Autodesk Inventor part; units mm, degrees
ref_plane "YZ Plane" through (0, 0, 0) normal (1, 0, 0) x (0, 1, 0)
ref_plane "XZ Plane" through (0, 0, 0) normal (0, 1, 0) x (-1, 0, 0)
ref_plane "XY Plane" through (0, 0, 0) normal (0, 0, 1) x (1, 0, 0)
sketch "Sketch1" plane through (0, 0, 0) normal (0, 0, 1) x (1, 0, 0)
  circle A0 centre (0, 0) radius 12.35
  circle A1 centre (7.4246, 7.4246) radius 12.2
  line L0 (-13.413, -13.413) -> (25.4094, 25.4094) construction
  line L1 (-10.6165, 0) -> (15.2552, 0) construction
  line L2 (7.4246, 7.4246) -> (15.8638, 6.41) construction
  line L3 (16.6649, 18.5138) -> (22.6753, 24.5242) construction
  circle A2 centre (15.8638, 6.41) radius 1.5
  line L4 (7.4246, 7.4246) -> (-1.0146, 8.4392) construction
  circle A3 centre (-1.0146, 8.4392) radius 1.5
  line L5 (0, 0) -> (-1.0146, 8.4392) construction
  line L6 (0, 0) -> (1.0146, -8.4392) construction
  circle A4 centre (1.0146, -8.4392) radius 1.5
  circle A5 centre (-9.8288, -9.8288) radius 12.2
  line L7 (-5.2409, -11.1828) -> (0, 0)
  point P0 (11.6813, -4.0087)
  point P1 (-0.7603, -1.6223)
  dimension "d0" = 24.7
  dimension "d1" = 24.4
  dimension "d2" = 0
  dimension "d3" = 45
  dimension "d4" = 0
  dimension "d5" = 10.5
  dimension "d20" = 8.5
  dimension "d21" = 3
  dimension "d22" = 3
  dimension "d23" = 3
  dimension "d24" = 24.4
  dimension "d25" = 24.4
  dimension "d26" = 4.5
extrude "Extrusion1" add sketch "Sketch1" along normal blind 3 contours A0 A5 A4 L7 A1 | A0 L7 A5 A4
sketch "Sketch3" plane through (0, 0, 3) normal (0, 0, 1) x (1, 0, 0)
  circle A0 centre (0, 0) radius 12.35
  circle A1 centre (7.4246, 7.4246) radius 12.2
  line L0 (-13.413, -13.413) -> (25.4094, 25.4094) construction
  line L1 (-10.6165, 0) -> (15.2552, 0) construction
  line L2 (7.4246, 7.4246) -> (15.8638, 6.41) construction
  line L3 (16.6649, 18.5138) -> (22.6753, 24.5242) construction
  circle A2 centre (15.8638, 6.41) radius 1.5
  line L4 (7.4246, 7.4246) -> (-1.0146, 8.4392) construction
  circle A3 centre (-1.0146, 8.4392) radius 1.5
  line L5 (0, 0) -> (-1.0146, 8.4392) construction
  line L6 (0, 0) -> (1.0146, -8.4392) construction
  circle A4 centre (1.0146, -8.4392) radius 1.5
  circle A5 centre (-9.8288, -9.8288) radius 12.2
  line L7 (-5.2409, -11.1828) -> (0, 0)
  point P0 (11.6813, -4.0087)
  point P1 (-0.7603, -1.6223)
  point P2 (-0.7743, -1.6522)
  point P3 (2.1356, -7.4425)
  point P4 (2.3507, -9.1211)
  point P5 (2.146, -12.1621)
  dimension "d32" = 24.7
  dimension "d33" = 24.4
  dimension "d34" = 0
  dimension "d35" = 45
  dimension "d36" = 0
  dimension "d37" = 10.5
  dimension "d38" = 8.5
  dimension "d39" = 3
  dimension "d40" = 3
  dimension "d41" = 3
  dimension "d42" = 24.4
  dimension "d43" = 24.4
  dimension "d44" = 4.5
extrude "Extrusion3" add sketch "Sketch3" along normal blind 15.5 contours A0 A5 A4 L7 A1 | A4 A5 picked at (2.3363, -8.2121)
sketch "Sketch4" plane through (0, 0, 3) normal (0, 0, 1) x (1, 0, 0)
  line L0 (-2.1493, -8.7099) -> (-0.8017, -5.8346)
  line L1 (-0.8017, -5.8346) -> (2.3621, -5.5639)
  line L2 (2.3621, -5.5639) -> (4.1785, -8.1686)
  line L3 (4.1785, -8.1686) -> (2.8309, -11.0439)
  line L4 (2.8309, -11.0439) -> (-0.3329, -11.3146)
  line L5 (-0.3329, -11.3146) -> (-2.1493, -8.7099)
  point P0 (0, 0)
  point P1 (1.0146, -8.4392)
  dimension "d49" = 5.5
extrude "Extrusion4" cut sketch "Sketch4" along normal blind 2 and the other way blind 1
sketch "Sketch5" plane through (0, 0, 18.5) normal (0, 0, 1) x (1, 0, 0)
  circle A0 centre (0, 0) radius 12.35
  circle A1 centre (7.4246, 7.4246) radius 12.2
  line L0 (-13.413, -13.413) -> (25.4094, 25.4094) construction
  line L1 (-10.6165, 0) -> (15.2552, 0) construction
  line L2 (7.4246, 7.4246) -> (15.8638, 6.41) construction
  line L3 (16.6649, 18.5138) -> (22.6753, 24.5242) construction
  circle A2 centre (15.8638, 6.41) radius 1.5
  line L4 (7.4246, 7.4246) -> (-1.0146, 8.4392) construction
  circle A3 centre (-1.0146, 8.4392) radius 1.5
  line L5 (0, 0) -> (-1.0146, 8.4392) construction
  line L6 (0, 0) -> (1.0146, -8.4392) construction
  circle A4 centre (1.0146, -8.4392) radius 1.5
  circle A5 centre (-9.8288, -9.8288) radius 12.2
  line L7 (-5.2409, -11.1828) -> (0, 0)
  line L8 (-30.7591, -9.8288) -> (7.4246, 28.355)
  line L9 (7.4246, 28.355) -> (28.355, 7.4246)
  line L10 (28.355, 7.4246) -> (-9.8288, -30.7591)
  line L11 (-9.8288, -30.7591) -> (-30.7591, -9.8288)
  circle A6 centre (-9.8288, -9.8288) radius 14.8
  circle A7 centre (7.4246, 7.4246) radius 14.8
  point P0 (11.6813, -4.0087)
  point P1 (-0.7603, -1.6223)
  point P2 (2.146, -12.1621)
  point P3 (-12.1621, 2.146)
  point P4 (-4.0087, 11.6813)
  point P5 (0.6364, -20.294)
  point P6 (17.8898, -3.0406)
  point P7 (-3.0406, 17.8898)
  point P8 (-20.294, 0.6364)
  dimension "d54" = 24.7
  dimension "d55" = 24.4
  dimension "d56" = 0
  dimension "d57" = 45
  dimension "d58" = 0
  dimension "d59" = 10.5
  dimension "d60" = 8.5
  dimension "d61" = 3
  dimension "d62" = 3
  dimension "d63" = 3
  dimension "d64" = 24.4
  dimension "d65" = 24.4
  dimension "d66" = 4.5
  dimension "d67" = 14.8
  dimension "d68" = 14.8
  dimension "d69" = 29.6
  dimension "d70" = 14.8
extrude "Extrusion5" add sketch "Sketch5" against normal blind 18.5 contours A0 A7 A1 | A0 A6 L8 A7 | A7 L10 A6 A0 | A0 A5 A6
fillet "Fillet1" radius 3 1 edges at (-5.2409, -11.1828, 1.5)
fillet "Fillet2" radius 3 1 edges at (-0.7603, -1.6223, 9.25)
properties part number "Hiolder_26"
Geometry: final body of the model. Coordinates: model frame, mm. A direction names the side the tool comes from. Give positions to 0.01 mm unless a question says otherwise; leave off trailing zeros. Write each loop counter-clockwise with the first axis right and the second up, starting at its lowest first coordinate (ties: lowest second). Pieces come first, ordered by that corner, then holes.
(1) First-contact query: P1, Ø4, axis at y = -15, z = 9, coming from the +X side; P2, Ø5, axis at x = 10.5, z = 2.5, coming from the -Y side; P3, Ø5, axis at x = -0.5, y = -10, coming from the +Z side. Flat tips, straight axial feed; report the tip coordinate or a pass-through.
(2) Mould query, pull axis X, two halves, no side actions, for faces 1 (the flat face through (9.38, -11.55, 9.38)), 2 (the flat face through (-11.79, 9.14, 9.38)), 3 (the cylindrical face through (-9.326, 8.096, 9.38)). Classes: released by +X, released by -X, zero draft, split by the parting line, or undercut.
(3) Access query for faces 4 (the flat face through (0, -7, 2)), 5 (the cylindrical face through (1.047, -3.144, 7.065)), 6 (the flat face through (2, -5, 18.5)), 7 (the flat face through (-1.485, -7.292, 2.493)). Directions: +Z, -Z, +X, -X, +Y, -Y. A direction counts if a zero-diameter tool reaches every point of the face in a straight line with its end or side. Return the directions, or none.
(4) Cut plane B-B, the plane x = 19. Return loops of the section in (y, z).
(5) Ray query, line 1 (Y direction, x = 0.5, z = 14.5); line 2 (Y direction, x = 4.5, z = 1); line 3 (X direction, y = 18.5, z = 10.25). Return the intervals inside material, ascending.
(6) Cut plane C-C, the plane y = -4. Return loops of the section in (x, z), then the cut area to 3 significant figures.
(7) Cut plane A-A, the plane y = -21. Return loops of the section in (x, z).
Values follow:
1. P1: stops at x = 7.93
1. P2: stops at y = -12.93
1. P3: stops at z = 3
2. face 1: released by +X
2. face 2: released by -X
2. face 3: undercut
3. face 4: none
3. face 5: +Z, -Z
3. face 6: +Z, +X, -X, +Y, -Y
3. face 7: +Z
4. outline: (-1.8, 0) - (3.57, 0) - (3.57, 18.5) - (-1.8, 18.5) - close; (11.28, 0) - (16.65, 0) - (16.65, 18.5) - (11.28, 18.5) - close
5. line 1: y = -20.43 to -16.32, -3.34 to -3.09, 17.47 to 20.5
5. line 2: y = -16.43 to -4.42, 19.27 to 21.93
5. line 3: x = -2.39 to 2.31, 12.54 to 17.24
6. outline: (-23.43, 0) - (-20.55, 0) - (-20.55, 18.5) - (-23.43, 18.5) - close; (-1.7, 0) - (3.14, 0) - (3.14, 18.5) - (0.89, 18.5) - (0.89, 3) - (-1.7, 3) - close; (11.7, 0) - (16.93, 0) - (16.93, 18.5) - (11.7, 18.5) - close
6. area: 200 mm2
7. outline: (-19.54, 0) - (-14.73, 0) - (-14.73, 18.5) - (-19.54, 18.5) - close; (-4.93, 0) - (-0.12, 0) - (-0.12, 18.5) - (-4.93, 18.5) - close
